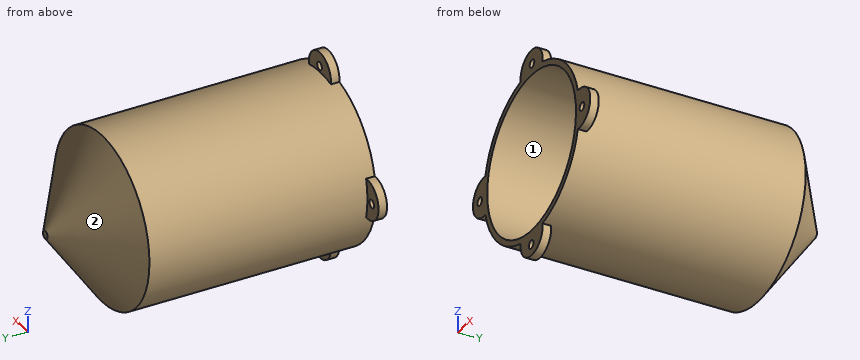
from build123d import *

# Parameters (mm, degrees)
SKETCH1_R                 = 30
BOSS_EXTRUDE1_DEPTH       = 100
CHAMFER1_SIZE             = 20
CHAMFER1_SIZE2            = 28.562960135
SHELL1_T                  = -2
BOSS_EXTRUDE2_DEPTH       = 3
F_1_0MM_DOWEL_HOLE1_D     = 2.9
F_1_0MM_DOWEL_HOLE1_DEPTH = 9.128752102
F_1_0MM_DOWEL_HOLE1_TIP   = 0.871247898


with BuildPart() as part:
    # Sketch1 → Boss-Extrude1 (new body)
    with BuildSketch(Plane(origin=(0, 0, 0), x_dir=(1, 0, 0), z_dir=(0, 1, 0))):
        with Locations(Location((0, 0, 0), (0, 0, 270))):
            Circle(SKETCH1_R)
    extrude(amount=BOSS_EXTRUDE1_DEPTH)

    # Chamfer1
    chamfer1_edges = [part.edges().sort_by_distance(p)[0] for p in [
        (0, 100, -30),
    ]]
    chamfer1_side = [part.faces().sort_by_distance(p)[0] for p in [
        (0, 50, -30),
    ]]
    chamfer(chamfer1_edges, length=CHAMFER1_SIZE, length2=CHAMFER1_SIZE2, reference=chamfer1_side[0])

    # Shell1
    shell1_openings = [part.faces().sort_by_distance(p)[0] for p in [
        (0, 0, 0),
    ]]
    offset(amount=SHELL1_T, openings=shell1_openings, kind=Kind.INTERSECTION)

    # Sketch2 → Boss-Extrude2 (add)
    with BuildSketch(Plane.XZ):
        with BuildLine():
            ThreePointArc((29.183333333, -6.952197894), (37, 0), (29.183333333, 6.952197894))
            ThreePointArc((29.183333333, 6.952197894), (29.795133831, 3.5), (30, 0))
            ThreePointArc((30, 0), (29.795133831, -3.5), (29.183333333, -6.952197894))
        make_face()
        with BuildLine():
            ThreePointArc((-6.952197894, 29.183333333), (0, 30), (6.952197894, 29.183333333))
            ThreePointArc((6.952197894, 29.183333333), (0, 37), (-6.952197894, 29.183333333))
        make_face()
        with BuildLine():
            ThreePointArc((-29.183333333, -6.952197894), (-30, 0), (-29.183333333, 6.952197894))
            ThreePointArc((-29.183333333, 6.952197894), (-37, 0), (-29.183333333, -6.952197894))
        make_face()
        with BuildLine():
            ThreePointArc((-6.952197894, -29.183333333), (0, -37), (6.952197894, -29.183333333))
            ThreePointArc((6.952197894, -29.183333333), (0, -30), (-6.952197894, -29.183333333))
        make_face()
    extrude(amount=-BOSS_EXTRUDE2_DEPTH)

    # Ø1.0mm Dowel Hole1
    with Locations(Plane(origin=(0.238867715, 0, 32.008273773), x_dir=(0, 0, -1), z_dir=(0, -1, 0))):
        with Locations((0, 0), (32.167518916, 31.530538344), (64.972018405, -0.47773543), (32.326764059, -32.963744633)):
            Hole(F_1_0MM_DOWEL_HOLE1_D / 2, depth=F_1_0MM_DOWEL_HOLE1_DEPTH)
            with Locations((0, 0, -(F_1_0MM_DOWEL_HOLE1_DEPTH + F_1_0MM_DOWEL_HOLE1_TIP / 2))):  # 118° drill point
                Cone(0, F_1_0MM_DOWEL_HOLE1_D / 2, F_1_0MM_DOWEL_HOLE1_TIP, mode=Mode.SUBTRACT)


solid = part.part
The model under review builds one solid part; all positions refer to its coordinate system, in mm. Face numbers are marked on the shaded views. Round coordinates to 2 decimals unless told otherwise and drop trailing zeros. Write each loop counter-clockwise with the first axis right and the second up, starting at its lowest first coordinate (ties: lowest second). Pieces come first, ordered by that corner, then holes. Notation, with made-up numbers: M 2,66 L 45,66 A23 ccw 45,98 Z; hole C -27.5,-16 d6. An arc over 180 degrees is marked long. Answer as CSV lines item,"result". Start each with the question number.
Q1. Consider section A-A, the plane y = 47.5. Give the boundary of the cut face in (x, z).
Q2. Wall thickness on line 1 along Z through (x, y) = (26, 75); line 2 along X through (y, z) = (92, 2); line 3 along X through (y, z) = (32.5, 13): over which ranges is each line inside the solid? List them lowest first.
Q3. The part is to be moulded in two halves that separate along X. For the marked faces 1 and 2, say which applies: +X half, -X half, draft (parallel to the pull), parting line (faces both ways), or undercut.
Q4. Consider section B-B, the plane y = 82.5. Give the boundary of the cut face in (x, z), then the cut area to 3 significant figures.
Q5. Clearance check with flat-ended pins moving along their axes: P1, Ø0.5, axis at x = 0, z = 0, coming from the -Y side; P2, Ø5, axis at x = 4, y = 47, coming from the -Z side; P3, Ø6, axis at x = 8, z = -17, coming from the +Y side. State where each tip first meets the part, or that it passes through.
Result set:
1,outline,"C 0,0 d60; hole C 0,0 d56"
2,line 1,"z = -14.97 to -10.39, 10.39 to 14.97"
2,line 2,"x = -12.71 to -9.16, 9.16 to 12.71"
2,line 3,"x = -27.04 to -24.8, 24.8 to 27.04"
3,face 1,"undercut"
3,face 2,"parting line"
4,outline,"C 0,0 d52.86; hole C 0,0 d45.89"
4,area,"541 mm²"
5,P1,"stops at y = 98"
5,P2,"stops at z = -29.96"
5,P3,"stops at y = 89.95"
